Autodesk Inventor part; units mm, degrees
ref_plane "YZ Plane" through (0, 0, 0) normal (1, 0, 0) x (0, 1, 0)
ref_plane "XZ Plane" through (0, 0, 0) normal (0, 1, 0) x (-1, 0, 0)
ref_plane "XY Plane" through (0, 0, 0) normal (0, 0, 1) x (1, 0, 0)
sketch "Sketch1" plane through (0, 0, 0) normal (0, 1, 0) x (-1, 0, 0)
  line L0 (0, 0) -> (95.25, 0)
  line L1 (95.25, 0) -> (95.25, -260.35)
  line L2 (95.25, -260.35) -> (0, -260.35)
  line L3 (0, -260.35) -> (0, 0)
  circle A0 centre (77.8624, -6.35) radius 3.175
  circle A1 centre (77.8624, -25.4) radius 3.175
  circle A2 centre (52.4624, -6.35) radius 3.175
  circle A3 centre (52.4624, -25.4) radius 3.175
  circle A4 centre (27.0624, -6.35) radius 3.175
  circle A5 centre (27.0624, -25.4) radius 3.175
  circle A6 centre (77.8624, -228.6) radius 3.175
  circle A7 centre (77.8624, -254) radius 3.175
  circle A8 centre (52.4624, -228.6) radius 3.175
  circle A9 centre (52.4624, -254) radius 3.175
  circle A10 centre (27.0624, -228.6) radius 3.175
  circle A11 centre (27.0624, -254) radius 3.175
  line L4 (101.24, -208.719) -> (15.24, -208.719) construction
  line L5 (15.24, -208.719) -> (15.24, -37.719) construction
  line L6 (15.24, -37.719) -> (101.24, -37.719) construction
  line L7 (101.24, -37.719) -> (101.24, -208.719) construction
  line L8 (95.25, -211.894) -> (12.065, -211.894)
  line L9 (12.065, -211.894) -> (12.065, -34.544)
  line L10 (12.065, -34.544) -> (95.25, -34.544)
  dimension "d0" = 95.25
  dimension "d2" = 6.35
  dimension "d3" = 6.35
  dimension "d4" = 17.3876
  dimension "d7" = 19.05
  dimension "d10" = 25.4
  dimension "d15" = 25.4
  dimension "d18" = 25.4
  dimension "d21" = 222.25
  dimension "d22" = 6.35
  dimension "d54" = 86
  dimension "d55" = 177.35
  dimension "d56" = 171
  dimension "d57" = 3.175
  dimension "d58" = 34.544
  dimension "d59" = 3.175
  dimension "d60" = 12.065
extrude "Plate1" add sketch "Sketch1" along normal blind 3.048 contours L0 L1 L10 L9 L8 L2 L3
sketch "Sketch2" plane through (-3.048, 3.048, 0) normal (1, 0, 0) x (0, 1, 0)
  line L0 (0, -260.35) -> (0, 0)
  line L1 (0, 0) -> (-50.8, 0)
  line L2 (-50.8, 0) -> (-50.8, -260.35)
  line L3 (-50.8, -260.35) -> (0, -260.35)
edge flange "Flange1" height 50.8 angle 90 thickness 3.048 bend radius 3.048 thickness toward (1, 0, 0) relief tear relief width 3.048 relief depth 1.524 edges at (0, 0, -130.175) wall of the first edge with corners at (-3.048, 3.048, -260.35) (-3.048, 3.048, 0) (-3.048, -47.752, 0) (-3.048, -47.752, -260.35)
bend "Bend1"
corner "Corner1"
sketch "Sketch3" plane through (0, -47.752, 0) normal (1, 0, 0) x (0, 0, -1)
  circle A0 centre (87.2198, 37.9611) radius 3.175
  circle A1 centre (61.8198, 12.5611) radius 3.175
  line L0 (0, 0) -> (0, 44.704)
  line L1 (260.35, 0) -> (0, 0)
  circle A2 centre (99.9198, 12.5611) radius 3.175
  circle A3 centre (138.0198, 12.5611) radius 3.175
  circle A4 centre (176.1198, 12.5611) radius 3.175
  circle A5 centre (125.3198, 37.9611) radius 3.175
  circle A6 centre (163.4198, 37.9611) radius 3.175
  circle A7 centre (61.8198, 12.5611) radius 9.525
  circle A8 centre (176.1198, 12.5611) radius 9.525
  line L2 (61.8198, 3.0361) -> (176.1198, 3.0361)
  line L3 (0, 44.704) -> (260.35, 44.704)
  line L4 (260.35, 44.704) -> (260.35, 0)
  line L5 (54.3999, 6.5886) -> (0, 41.529)
  line L6 (184.6703, 8.3641) -> (201.5198, 41.529)
  line L7 (201.5198, 41.529) -> (260.35, 41.529)
  point P0 (0, 47.752)
  point P1 (178.7879, 44.704)
  dimension "d34" = 6.35
  dimension "d35" = 25.4
  dimension "d36" = 25.4
  dimension "d37" = 61.8198
  dimension "d40" = 38.1
  dimension "d47" = 38.1
  dimension "d61" = 6.35
  dimension "d62" = 6.35
  dimension "d64" = 3.175
  dimension "d65" = 3.175
  dimension "d66" = 25.4
extrude "Cut1" cut sketch "Sketch3" against normal blind 3.048 contours A0 | A1 | L0 L5 A7 L2 A8 L6 L7 L4 L1 | A2 | A3 | A4 | A5 | A6
fillet "Fillet1" radius 3.175 8 edges at (-95.25, 1.524, 0) (-95.25, 1.524, -34.544) (-12.065, 1.524, -34.544) (-95.25, 1.524, -211.894) (-12.065, 1.524, -211.894) (-95.25, 1.524, -260.35) (-1.524, -6.223, -201.5198) (-1.524, -6.223, 0)
equation "\"d65\" = d64"
equation "\"d52\" = Thickness"
equation "\"d23\" = Thickness"
equation "\"d24\" = BendReliefWidth"
equation "\"d25\" = BendReliefDepth"
equation "\"d26\" = MinimumRemnant"
equation "\"d27\" = TransitionRadius"
equation "\"d30\" = BendRadius"
equation "\"d31\" = CornerReliefSize"
equation "\"d32\" = GapSize"
equation "\"d33\" = JacobiRadiusSize"
equation "\"BendRadius\" = Thickness"
equation "\"BendReliefWidth\" = Thickness"
equation "\"BendReliefDepth\" = 0.5 * Thickness"
equation "\"CornerReliefSize\" = 4 * Thickness"
equation "\"MinimumRemnant\" = 2 * Thickness"
equation "\"TransitionRadius\" = BendRadius"
equation "\"JacobiRadiusSize\" = BendRadius"
equation "\"GapSize\" = Thickness"
properties part number "MainDriveMotorToPlateConnector"
Here's how the part is built. I have some questions about the finished solid (model axes, mm). A direction names the side the tool comes from. Round coordinates to 2 decimals unless told otherwise and drop trailing zeros. Loops run counter-clockwise (first coordinate to the right, second up) from the corner with the lowest first, then second, coordinate; pieces in that order, holes last. Notation, with made-up numbers: (33.25, 57.25) - (68.25, 57.25) arc R22 ccw to (68.25, 96.25) - close; hole circle Ø8 at (-23.75, 9). An arc over 180 degrees is marked (long way). One line per question, with ' | ' between items. Start each with the question number.
Q1. I want a section at B-B (x = -42.5). Write out the boundary of the cut face in (y, z), then the cut area to 3 significant figures.
Q2. I want a section at C-C (z = -50.5). Write out the boundary of the cut face in (x, y) (3 decimals).
Q3. I want a section at A-A (z = -254). Write out the boundary of the cut face in (x, y), then the cut area to 3 significant figures.
Q4. I want a section at D-D (z = -6.35). Write out the boundary of the cut face in (x, y), then the cut area to 3 significant figures.
Q5. Will these pins go through, and if not, where does the flat tip stop? pin 1 (2 mm diameter, centred on y = -8, z = -148, fed in from -X); pin 2 (8.5 mm diameter, centred on x = -27.06, z = -6.35, fed in from -Y).
Q6. For faces 1 (the flat face through (0, -20, -128)), 2 (the flat face through (-10, 0, -157)), which set-ups out of +Z, -Z, +X, -X, +Y, -Y let a thin tool reach every point of the face, with its end or its side?
Q7. Please list where these lines run through material, in increasing order: line 1 (X direction, y = -8, z = -65); line 2 (Y direction, x = -57, z = -17); line 3 (Y direction, x = -5, z = -144). Write a range as [from, to].
Q8. We'd pull the mould along Y, two halves only. Please class faces 3 (the cylindrical face through (-51.77, 1.5, -250.9)), 4 (the cylindrical face through (-1.5, -8.84, -90.25)), 5 (the cylindrical face through (-1.5, -11.01, -166.35)), 6 (the cylindrical face through (-1.503, -43.314, -181.094)): +Y half, -Y half, draft (parallel to the pull), parting line (faces both ways), or undercut.
Response values:
1) outline: (0, -260.35) - (3.05, -260.35) - (3.05, -211.89) - (0, -211.89) - close; (0, -34.54) - (3.05, -34.54) - (3.05, 0) - (0, 0) - close | area: 253 mm²
2) outline: (-12.065, 0) - (-6.096, 0) arc R3.048 cw to (-3.048, -3.048) - (-3.048, -38.659) - (0, -38.659) - (0, -3.048) arc R6.096 ccw to (-6.096, 3.048) - (-12.065, 3.048) - close
3) outline: (-95.25, 0) - (-81.04, 0) - (-81.04, 3.05) - (-95.25, 3.05) - close; (-74.69, 0) - (-55.64, 0) - (-55.64, 3.05) - (-74.69, 3.05) - close; (-49.29, 0) - (-30.24, 0) - (-30.24, 3.05) - (-49.29, 3.05) - close; (-23.89, 0) - (-6.1, 0) arc R3.05 cw to (-3.05, -3.05) - (-3.05, -6.22) - (0, -6.22) - (0, -3.05) arc R6.1 ccw to (-6.1, 3.05) - (-23.89, 3.05) - close | area: 245 mm²
4) outline: (-95.25, 0) - (-81.04, 0) - (-81.04, 3.05) - (-95.25, 3.05) - close; (-74.69, 0) - (-55.64, 0) - (-55.64, 3.05) - (-74.69, 3.05) - close; (-49.29, 0) - (-30.24, 0) - (-30.24, 3.05) - (-49.29, 3.05) - close; (-23.89, 0) - (-6.1, 0) arc R3.05 cw to (-3.05, -3.05) - (-3.05, -10.3) - (0, -10.3) - (0, -3.05) arc R6.1 ccw to (-6.1, 3.05) - (-23.89, 3.05) - close | area: 258 mm²
5) pin 1: stops at x = -3.05 | pin 2: stops at y = 0
6) face 1: +Z, -Z, +X, +Y, -Y | face 2: +Z, -Z, -X, -Y
7) line 1: x = [-3.05, 0] | line 2: y = [0, 3.05] | line 3: y = [-0.2, 2.95]
8) face 3: draft | face 4: undercut | face 5: undercut | face 6: -Y half
